from build123d import *

# Parameters (mm, degrees)
SKETCH1_W           = 200
SKETCH1_H           = 200
BOSS_EXTRUDE1_DEPTH = 5
SKETCH8_W           = 15
SKETCH8_H           = 7
CUT_EXTRUDE4_DEPTH  = 142.509716981
BOSS_EXTRUDE2_DEPTH = 200
CUT_EXTRUDE6_REACH  = 143.774
SKETCH10_W          = 45.2
SKETCH10_H          = 15.4
CUT_EXTRUDE7_START  = -0.7
CUT_EXTRUDE7_DEPTH  = 3.6
SKETCH12_R          = 2.1
CUT_EXTRUDE8_DEPTH  = 142.774468788
CUT_EXTRUDE9_START  = -200
SKETCH13_W          = 21.4
SKETCH13_H          = 7.5
CUT_EXTRUDE9_DEPTH  = 200
CUT_EXTRUDE12_DEPTH = 3
FILLET1_R           = 8
CHAMFER1_SIZE2      = 6
CHAMFER1_SIZE       = 3


with BuildPart() as part:
    # Sketch1 → Boss-Extrude1 (new body)
    with BuildSketch(Plane(origin=(0, 0, 0), x_dir=(1, 0, 0), z_dir=(0, 1, 0))):
        Rectangle(SKETCH1_W, SKETCH1_H)
    extrude(amount=BOSS_EXTRUDE1_DEPTH)

    # Sketch8 → Cut-Extrude4 (cut, through all)
    with BuildSketch(Plane(origin=(0, 5, 0), x_dir=(1, 0, 0), z_dir=(0, 1, 0))):
        with Locations((-77.5, 32.5)):
            Rectangle(SKETCH8_W, SKETCH8_H)
    extrude(amount=-CUT_EXTRUDE4_DEPTH, mode=Mode.SUBTRACT)

    # Sketch9 → Boss-Extrude2 (add)
    with BuildSketch(Plane(origin=(100, 0, 0), x_dir=(0, 0, -1), z_dir=(1, 0, 0))):
        Polygon((-100, 5), (-3, 15), (-3, 5), align=None)
        Polygon((3, 5), (100, 5), (3, 15), align=None)
    extrude(amount=-BOSS_EXTRUDE2_DEPTH)

    # Cut-Extrude6: up to this plane
    cut_extrude6_end = Plane(origin=(-197.514101544, 5, -100), z_dir=(0, 0.9947279261542806, -0.1025492707375547))
    # Sketch10 → Cut-Extrude6 (cut, up to the surface)
    with BuildSketch(Plane(origin=(0, 5, 0), x_dir=(1, 0, 0), z_dir=(0, 1, 0)), mode=Mode.PRIVATE) as cut_extrude6_sk1:
        with Locations((-77.4, 32.5)):
            Rectangle(SKETCH10_W, SKETCH10_H)
    cut_extrude6_tool1 = split(extrude(cut_extrude6_sk1.sketch, amount=CUT_EXTRUDE6_REACH, mode=Mode.PRIVATE), bisect_by=cut_extrude6_end, keep=Keep.BOTH, mode=Mode.PRIVATE)
    add(cut_extrude6_tool1.solids().sort_by_distance((-77.4, 5, -32.5))[0], mode=Mode.SUBTRACT)

    # Sketch11 → Cut-Extrude7 (cut)
    with BuildSketch(Plane(origin=(0, 5, 0), x_dir=(1, 0, 0), z_dir=(0, 1, 0)).offset(CUT_EXTRUDE7_START)):
        Polygon((-92.5, 36.772391992), (-96.2, 34.636195996), (-96.2, 30.363804004), (-92.5, 28.227608008), (-88.8, 30.363804004), (-88.8, 34.636195996), align=None)
        Polygon((-62.5, 36.772391992), (-66.2, 34.636195996), (-66.2, 30.363804004), (-62.5, 28.227608008), (-58.8, 30.363804004), (-58.8, 34.636195996), align=None)
    extrude(amount=-CUT_EXTRUDE7_DEPTH, mode=Mode.SUBTRACT)

    # Sketch12 → Cut-Extrude8 (cut, through all)
    with BuildSketch(Plane(origin=(0, 5, 0), x_dir=(1, 0, 0), z_dir=(0, 1, 0))):
        with Locations(Location((-92.5, 32.5, 0), (0, 0, 270))):
            Circle(SKETCH12_R)
        with Locations(Location((-62.5, 32.5, 0), (0, 0, 270))):
            Circle(SKETCH12_R)
    extrude(amount=-CUT_EXTRUDE8_DEPTH, mode=Mode.SUBTRACT)

    # Sketch13 → Cut-Extrude9 (cut)
    with BuildSketch(Plane.ZY.offset(100).offset(CUT_EXTRUDE9_START)):
        with Locations((0, 8.75)):
            Rectangle(SKETCH13_W, SKETCH13_H)
    extrude(amount=CUT_EXTRUDE9_DEPTH, mode=Mode.SUBTRACT)

    # Sketch16 → Cut-Extrude12 (cut)
    with BuildSketch(Plane.XZ):
        Polygon((-85, -29), (-85, -13), (-55, -13), (-55, -21), (-70, -21), (-70, -29), align=None)
    extrude(amount=-CUT_EXTRUDE12_DEPTH, mode=Mode.SUBTRACT)

    # Fillet1
    fillet1_edges = [part.edges().sort_by_distance(p)[0] for p in [
        (-70, 1.5, -21),
        (-85, 1.5, -13),
    ]]
    fillet(fillet1_edges, radius=FILLET1_R)

    # Chamfer1
    chamfer1_edges = [part.edges().sort_by_distance(p)[0] for p in [
        (-55, 0, -17),
    ]]
    chamfer1_side = [part.faces().sort_by_distance(p)[0] for p in [
        (-55, 0.06, -17),
    ]]
    chamfer(chamfer1_edges, length=CHAMFER1_SIZE - 0.0001, length2=CHAMFER1_SIZE2 - 0.0001, reference=chamfer1_side[0])  # a hair under: the kernel refuses the full size


solid = part.part
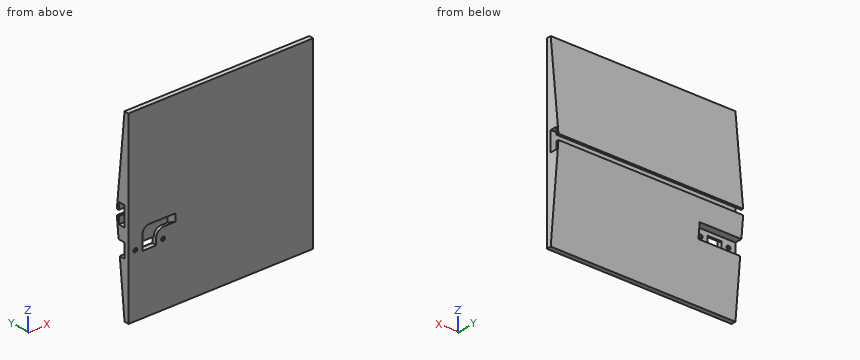
Could you check a few things on this model? Use its own coordinates, in mm. Coordinates: 2 decimals unless noted, no trailing zeros. Order: outer loops, then holes, each group sorted by start corner. A loop starts at its lowest first (then second) coordinate and runs counter-clockwise, first axis right, second up. Notation, with made-up numbers: (8, 1) -> (17, 1) arc R27 cw to (17, 40) -> close; hole circle Ø3 at (-15, 16). An arc over 180 degrees is marked (long way). One line per item, written item: value. Start each with the question number.
1) Imagine slicing it at C-C on z = 18. List the corners of the cut face in (x, y) for me.
2) I'm going to push flat-ended pins straight in: pin 1 (2.5 mm diameter, centred on y = 9, z = -30, fed in from -X); pin 2 (2 mm diameter, centred on x = -66.5, z = -33.5, fed in from +Y). Where does each tip first touch, or does it pass through?
3) Imagine slicing it at B-B on x = 0.5. List the corners of the cut face in (y, z) for me.
4) Imagine slicing it at D-D on z = 71. List the corners of the cut face in (x, y) for me, plus the area to 3 significant figures.
5) If I drill on L1, parallel to X at y = 0.5, z = -32.5; L2, parallel to Z at x = -81.5, y = 3.25; L3, parallel to X at y = 5.25, z = -28, over which ranges is the centre line in solid material (lowest first)? Write a range as [from, to].
6) Imagine slicing it at A-A on y = 7.5. List the corners of the cut face in (x, z) for me, plus the area to 3 significant figures.
Answer list:
1. outline: (-100, 0) -> (100, 0) -> (100, 13.45) -> (-100, 13.45) -> close
2. pin 1: stops at x = -54.8
2. pin 2: stops at y = 5
3. outline: (0, -100) -> (5, -100) -> (15, -3) -> (12.5, -3) -> (12.5, -10.7) -> (5, -10.7) -> (5, 10.7) -> (12.5, 10.7) -> (12.5, 3) -> (15, 3) -> (5, 100) -> (0, 100) -> close
4. outline: (-100, 0) -> (100, 0) -> (100, 7.99) -> (-100, 7.99) -> close
4. area: 1,600 mm2
5. L1: x = [-100, -94.6], [-90.4, -85], [-70, -64.6], [-60.4, 100]
5. L2: z = [-100, -36], [-29, 100]
5. L3: x = [-54.8, 100]
6. outline: (-100, -75.75) -> (100, -75.75) -> (100, -10.7) -> (-100, -10.7) -> (-100, -24.8) -> (-54.8, -24.8) -> (-54.8, -40.2) -> (-100, -40.2) -> close; (-100, 10.7) -> (100, 10.7) -> (100, 75.75) -> (-100, 75.75) -> close
6. area: 25,300 mm2
